Geometry: final body of the model. Coordinates: model frame, mm. Face numbers are marked on the shaded views. A direction names the side the tool comes from. Round coordinates to 2 decimals unless told otherwise and drop trailing zeros. Write each loop counter-clockwise with the first axis right and the second up, starting at its lowest first coordinate (ties: lowest second). Pieces come first, ordered by that corner, then holes. Notation, with made-up numbers: M 76,68.25 L 91,68.25 A15 cw 91,88.25 Z; hole C 32,25.5 d2. An arc over 180 degrees is marked long. Answer as CSV lines item,"result". Start each with the question number.
Q1. Ray query, probe 1 along Z at (x, y) = (0, 2.25); probe 2 along X at (y, z) = (4.25, 0); probe 3 along X at (y, z) = (5.25, 55). Return the intervals inside material, ascending.
Q2. Section query D-D on y = 13. Output: boundary loops of the cut face in (x, z).
Q3. Section query B-B on z = 55. Output: boundary loops of the cut face in (x, y) (1 decimal).
Q4. Section query A-A on y = 2.25. Output: boundary loops of the cut face in (x, z).
Q5. Mould query, pull axis Z, two halves, no side actions, for the marked faces 1, 2 and 3. Classes: pulls with the +Z half, pulls with the -Z half, needs draft (parallel to the pull), parting line crosses it, or undercut.
Q6. Reachability of the marked faces 4, 5 and 6 from +Z, -Z, +X, -X, +Y, -Y: full face, straight path, thin tool, end or side. Return the list, or none.
Q7. First-contact query: pin 1 (12 mm diameter, centred on x = 13, z = -42.5, fed in from +Y); pin 2 (6 mm diameter, centred on y = 24, z = -24, fed in from +X); pin 3 (4 mm diameter, centred on x = -46, y = 6.5, fed in from +Z); pin 4 (1.5 mm diameter, centred on x = -29.5, y = 19.5, fed in from -Z). Flat tips, straight axial feed; report the tip coordinate or a pass-through.
Q8. Section query C-C on x = -55. Output: boundary loops of the cut face in (y, z) (1 decimal), and give its area (3 significant figures).
Autodesk Inventor part; units mm, degrees
ref_plane "YZ Plane" through (0, 0, 0) normal (1, 0, 0) x (0, 1, 0)
ref_plane "XZ Plane" through (0, 0, 0) normal (0, 1, 0) x (-1, 0, 0)
ref_plane "XY Plane" through (0, 0, 0) normal (0, 0, 1) x (1, 0, 0)
sketch "Sketch1" plane through (0, 0, 0) normal (0, 1, 0) x (-1, 0, 0)
  circle A0 centre (0, 0) radius 55
  dimension "d0" = 110
extrude "Extrusion1" add sketch "Sketch1" along normal blind 10
sketch "Sketch2" plane through (0, 10, 0) normal (0, 1, 0) x (1, 0, 0)
  circle A0 centre (0, 0) radius 50
  dimension "d3" = 100
extrude "Extrusion2" add sketch "Sketch2" along normal blind 10
chamfer "Chamfer1" distance 10 angle 45 1 edges at (-50, 20, 0)
sketch "Sketch3" plane through (0, 20, 0) normal (0, 1, 0) x (1, 0, 0)
  circle A0 centre (0, 0) radius 40
  dimension "d9" = 80
extrude "Extrusion3" add sketch "Sketch3" along normal blind 10
sketch "Sketch4" plane through (0, 10, 0) normal (0, 1, 0) x (1, 0, 0)
  circle A0 centre (0, 0) radius 60
  dimension "d12" = 120
extrude "Extrusion4" add sketch "Sketch4" against normal blind 10
sketch "Sketch5" plane through (0, 10, 0) normal (0, 1, 0) x (1, 0, 0)
  circle A0 centre (0, 55) radius 3.625
  circle A1 centre (0, 0) radius 60
  circle A2 centre (-55, 0) radius 3.625
  circle A3 centre (0, -55) radius 3.625
  circle A4 centre (55, 0) radius 3.625
  dimension "d15" = 7.25
  dimension "d16" = 55
  dimension "d19" = 360
extrude "Extrusion5" cut sketch "Sketch5" against normal blind 2.1735 draft -45 contours A0 | A2 | A3 | A4
sketch "Sketch6" plane through (0, 10, 0) normal (0, 1, 0) x (1, 0, 0)
  circle A0 centre (0, 55) radius 1.4515
  circle A1 centre (0, 0) radius 60
  circle A2 centre (-55, 0) radius 1.4515
  circle A3 centre (0, -55) radius 1.4515
  circle A4 centre (55, 0) radius 1.4515
  dimension "d23" = 2.903
  dimension "d24" = 55
  dimension "d27" = 360
extrude "Extrusion6" cut sketch "Sketch6" against normal through all contours A0 | A2 | A3 | A4
sketch "Sketch7" plane through (0, 30, 0) normal (0, 1, 0) x (1, 0, 0)
  line L0 (15, 7.5) -> (-15, 7.5)
  line L1 (-15, 7.5) -> (-15, -7.5)
  line L2 (-15, -7.5) -> (15, -7.5)
  line L3 (15, -7.5) -> (15, 7.5)
  line L4 (15, 7.5) -> (-15, -7.5) construction
  line L5 (-15, 7.5) -> (15, -7.5) construction
  point P0 (0, 0)
  dimension "d31" = 30
  dimension "d32" = 15
extrude "Extrusion7" cut sketch "Sketch7" against normal through all
sketch "Sketch8" plane through (0, 30, 0) normal (0, 1, 0) x (1, 0, 0)
  circle A0 centre (-23, 0) radius 1.4515
  circle A1 centre (0, 0) radius 40
  circle A2 centre (23, 0) radius 1.4515
  dimension "d35" = 2.903
  dimension "d36" = 23
  dimension "d39" = 360
extrude "Extrusion8" cut sketch "Sketch8" against normal through all contours A0 | A2
properties part number "base 1"
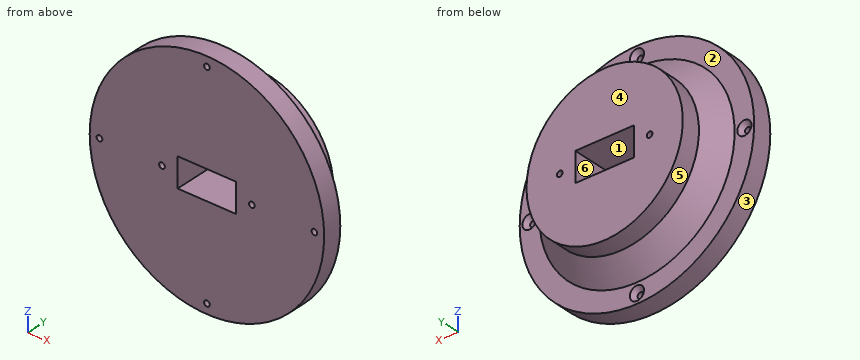
Entries:
1,probe 1,"z = -60 to -56.45, -53.55 to -7.5, 7.5 to 53.55, 56.45 to 60"
1,probe 2,"x = -60 to -56.45, -53.55 to -24.45, -21.55 to -15, 15 to 21.55, 24.45 to 53.55, 56.45 to 60"
1,probe 3,"x = -23.98 to -1.45, 1.45 to 23.98"
2,outline,"C 0,0 d94; hole C -23,0 d2.9; hole M -15,-7.5 L 15,-7.5 L 15,7.5 L -15,7.5 Z; hole C 23,0 d2.9"
3,outline,"M -24,0 L -1.5,0 L -1.5,7.8 L -3.6,10 L -24,10 Z; M 1.5,0 L 24,0 L 24,10 L 3.6,10 L 1.5,7.8 Z"
4,outline,"C 0,0 d120; hole C -55,0 d2.9; hole C -23,0 d2.9; hole M -15,-7.5 L 15,-7.5 L 15,7.5 L -15,7.5 Z; hole C 0,-55 d2.9; hole C 0,55 d2.9; hole C 23,0 d2.9; hole C 55,0 d2.9"
5,face 1,"undercut"
5,face 2,"needs draft"
5,face 3,"parting line crosses it"
6,face 4,"+Z, -Z, +X, -X, +Y"
6,face 5,"+Y"
6,face 6,"+Y, -Y"
7,pin 1,"stops at y = 30"
7,pin 2,"stops at x = 34.04"
7,pin 3,"stops at z = 40.79"
7,pin 4,"stops at z = -29.07"
8,outline,"M 0,-24 L 10,-24 L 10,-3.6 L 7.8,-1.5 L 0,-1.5 Z; M 0,1.5 L 7.8,1.5 L 10,3.6 L 10,24 L 0,24 Z"
8,area,"446 mm^2"
